Could you check a few things on this model? Use its own coordinates, in mm. A direction names the side the tool comes from. Give positions to 0.01 mm unless a question says otherwise; leave off trailing zeros. Loops run counter-clockwise (first coordinate to the right, second up) from the corner with the lowest first, then second, coordinate; pieces in that order, holes last. Notation, with made-up numbers: (15.5, 18) - (31.5, 18) arc R15 ccw to (31.5, 29) - close; hole circle Ø4 at (61, 44.25). An arc over 180 degrees is marked (long way). Use CSV: the item, a comma, the result in double quotes.
from build123d import *

# Parameters (mm, degrees)
OTHER_START              = -500
OTHER_2_DEPTH            = 1000
CUT_EXTRUDE_3_DEPTH      = 534.686237409
CUT_EXTRUDE_3_DEPTH_BACK = 534.686237409
SKETCH_11_R              = 3.5


# Read off the part's stored shape, not the designer's step: Элемент по сечениям сгиба2
with BuildPart() as part:
    # Other 2 outline → Other 2 (new body)
    with BuildSketch(Plane.YZ.offset(OTHER_START)):
        with BuildLine():
            Line((0, -111), (150, -111))
            Line((150, -111), (150, -108))
            Line((150, -108), (0, -108))
            ThreePointArc((0, -108), (-108, 0), (0, 108))
            Line((0, 108), (150, 108))
            Line((150, 108), (150, 111))
            Line((150, 111), (0, 111))
            ThreePointArc((0, 111), (-111, 0), (0, -111))
        make_face()
    extrude(amount=OTHER_2_DEPTH)

    # Эскиз11 → Вырез-Вытянуть3 (cut, two sides: drawn at the far end of the back side and taken through both)
    with BuildSketch(Plane.XY.offset(-CUT_EXTRUDE_3_DEPTH_BACK)):
        with Locations((450, 75)):
            Circle(SKETCH_11_R)
        with Locations((300, 75)):
            Circle(SKETCH_11_R)
        with Locations((150, 75)):
            Circle(SKETCH_11_R)
        with Locations((0, 75)):
            Circle(SKETCH_11_R)
        with Locations((-150, 75)):
            Circle(SKETCH_11_R)
        with Locations((-300, 75)):
            Circle(SKETCH_11_R)
        with Locations((-450, 75)):
            Circle(SKETCH_11_R)
    extrude(amount=CUT_EXTRUDE_3_DEPTH + CUT_EXTRUDE_3_DEPTH_BACK, mode=Mode.SUBTRACT)


solid = part.part
1) Suppose I cut it at B-B (x = -425.5). Please give me the cut outline in (y, z), plus the area to 3 significant figures.
Answer below:
outline,"(0, -111) - (150, -111) - (150, -108) - (0, -108) arc R108 cw to (0, 108) - (150, 108) - (150, 111) - (0, 111) arc R111 ccw to start"
area,"1,930 mm2"
2) Suppose I cut it at D-D (y = -83). Please give me the cut outline in (x, z), plus the area to 3 significant figures.
Answer below:
outline,"(-500, -73.7) - (500, -73.7) - (500, -69.1) - (-500, -69.1) - close; (-500, 69.1) - (500, 69.1) - (500, 73.7) - (-500, 73.7) - close"
area,"9,200 mm2"
3) Which directions (+Z, -Z, +X, -X, +Y, -Y) give clear straight access to the entire face, cutting with the end or side of a thin tool? Please do faces 1 (the flat face through (-7, 74, 108)), 2 (the flat face through (-7, 76, 111)).
Answer below:
face 1,"+X, -X, +Y"
face 2,"+Z, +X, -X, +Y, -Y"
4) Suppose I cut it at A-A (y = 15). Please give me the cut outline in (x, z), plus the area to 3 significant figures.
Answer below:
outline,"(-500, -111) - (500, -111) - (500, -108) - (-500, -108) - close; (-500, 108) - (500, 108) - (500, 111) - (-500, 111) - close"
area,"6,000 mm2"
5) I need wall thicknesses on line 1 along Z through (x, y) = (-140, 50); line 2 along Z through (x, y) = (170.5, -64); line 3 along Y through (x, z) = (436, -24). Which ranges of each line are inside material? Lowest first, please.
Answer below:
line 1,"z = -111 to -108, 108 to 111"
line 2,"z = -90.69 to -86.99, 86.99 to 90.69"
line 3,"y = -108.37 to -105.3"
6) We'd pull the mould along Z, two halves only. Please class faces 3 (the flat face through (-500, -107, 17)), 4 (the flat face through (-7, 76, -108)), 5 (the flat face through (-7, 74, -111)), 6 (the cylindrical face through (-7, -107.974, -2.375)): +Z half, -Z half, draft (parallel to the pull), parting line (faces both ways), or undercut.
Answer below:
face 3,"draft"
face 4,"undercut"
face 5,"-Z half"
face 6,"undercut"
7) I'm going to push flat-ended pins straight in: P1, Ø2, axis at x = 195, y = -28.5, coming from the +Z side; P2, Ø6.5, axis at x = 150, y = 75, coming from the -Z side; P3, Ø3, axis at x = 328.5, z = -82.5, coming from the -Y side; P4, Ø1.5, axis at x = -322.5, z = 42.5, coming from the +Y side. Where does each tip first touch, or does it pass through?
Answer below:
P1,"stops at z = 107.54"
P2,"passes through"
P3,"stops at y = -75.89"
P4,"stops at y = -98.96"
8) Suppose I cut it at C-C (z = 0). Please give me the cut outline in (x, y).
Answer below:
outline,"(-500, -111) - (500, -111) - (500, -108) - (-500, -108) - close"
